The model under review builds one solid part; all positions refer to its coordinate system, in mm. A direction names the side the tool comes from. Give positions to 0.01 mm unless a question says otherwise; leave off trailing zeros. Loops run counter-clockwise (first coordinate to the right, second up) from the corner with the lowest first, then second, coordinate; pieces in that order, holes last. Notation, with made-up numbers: M -30,74.25 L 22,74.25 A30 ccw 22,106.25 Z; hole C 54.25,12 d9. An arc over 180 degrees is marked long. One line per item, written item: value. Start each with the question number.
Q1. We need section C-C on y = 109. Write out the cut boundary in (x, z), plus the area to 3 significant figures.
Q2. For faces 1 (the face through (-1.633, 6.439, -49.684)), 2 (the face through (-0.253, 116.165, -66.719)), 3 (the face through (4, 64, -60.458)), 4 (the face through (-1.633, 112.374, 15.653)), list the 3-axis set-ups (+Z, -Z, +X, -X, +Y, -Y) from which the entire face can be reached by the end or side of a thin tool; tool diameter is ignored.
Q3. For pin 1 (1.5 mm diameter, centred on y = 96.5, z = -54, fed in from +X); pin 2 (2.5 mm diameter, centred on x = -1.03, y = 12.7, fed in from +Z), all flat-tipped, find the tip position at first contact; note any pin that passes through.
Q4. To check wall thickness, follow line 1 along Z through (x, y) = (-2.5, 11.5); line 2 along Y through (x, z) = (2.75, 3); line 3 along X through (y, z) = (114, -67). State the ranges of each line that lie inside material, in increasing order. Write a range as from..to.
Q5. We need section B-B on z = 11. Write out the cut boundary in (x, y).
Q6. We need section A-A on y = 34. Write out the cut boundary in (x, z).
Q7. Mouldability with a two-part tool opening along X and no side actions: class faces 5 (the face through (-1.011, 13.703, -47.408)), 6 (the face through (-1, 63, -73.158)), 7 (the face through (-1.011, 113.95, -59.455)), 8 (the face through (5.323, 68, 10)) as released by +X, released by -X, zero draft, split by the parting line, or undercut.
Autodesk Inventor part; units mm, degrees
ref_plane "YZ Plane" through (0, 0, 0) normal (1, 0, 0) x (0, 1, 0)
ref_plane "XZ Plane" through (0, 0, 0) normal (0, 1, 0) x (-1, 0, 0)
ref_plane "XY Plane" through (0, 0, 0) normal (0, 0, 1) x (1, 0, 0)
sketch "Sketch1" plane through (0, 0, 0) normal (0, 1, 0) x (-1, 0, 0)
  line L0 (7.3766, 22.0919) -> (-5.3234, 22.0919)
  line L1 (-5.3234, 22.0919) -> (-5.3234, -73.1581)
  line L2 (-5.3234, -73.1581) -> (7.3766, -73.1581)
  line L3 (7.3766, -73.1581) -> (7.3766, 22.0919)
  point P0 (0, 0)
  dimension "d0" = 12.7
  dimension "d1" = 95.25
extrude "Extrusion1" add sketch "Sketch1" along normal blind 127
sketch "Sketch2" plane through (-7.3766, 0, 22.0919) normal (0, 0, 1) x (1, 0, 0)
  line L0 (12.7, 0) -> (12.7, 127)
  line L1 (12.7, 127) -> (0, 127)
  line L2 (0, 0) -> (12.7, 0)
  line L3 (0, 0) -> (0, 127)
  point P0 (7.3766, 0)
  point P1 (6.35, 114.3)
  point P2 (6.35, 12.7)
  dimension "d4" = 6.35
  dimension "d5" = 12.7
  dimension "d6" = 12.7
  dimension "d7" = 6.35
hole "Hole1" at (-1.0266, 114.3, 22.0919) at (-1.0266, 12.7, 22.0919) direction (0, 0, -1) diameter 4.0386 depth 12.7 tip angle 118
sketch "Sketch3" plane through (5.3234, 0, -73.1581) normal (0, 0, -1) x (-1, 0, 0)
  line L0 (0, 0) -> (12.7, 0)
  line L1 (12.7, 0) -> (12.7, 127)
  line L2 (0, 127) -> (12.7, 127)
  point P0 (5.3234, 0)
  point P1 (6.35, 114.3)
  point P2 (6.35, 12.7)
  dimension "d15" = 12.7
  dimension "d16" = 6.35
  dimension "d17" = 6.35
  dimension "d18" = 12.7
hole "Hole2" at (-1.0266, 114.3, -73.1581) at (-1.0266, 12.7, -73.1581) direction (0, 0, 1) diameter 4.0386 depth 12.7 tip angle 118
sketch "Sketch4" plane through (5.3234, 0, 22.0919) normal (1, 0, 0) x (0, 0, -1)
  line L0 (12.7, 120.65) -> (82.55, 120.65)
  line L1 (82.55, 120.65) -> (82.55, 6.35)
  line L2 (82.55, 6.35) -> (12.7, 6.35)
  line L3 (12.7, 6.35) -> (12.7, 120.65)
  line L4 (95.25, 127) -> (0, 127)
  line L5 (95.25, 0) -> (0, 0)
  line L6 (95.25, 0) -> (95.25, 127)
  line L7 (0, 0) -> (0, 127)
  point P0 (22.0919, 0)
  dimension "d26" = 6.35
  dimension "d27" = 6.35
  dimension "d28" = 12.7
  dimension "d29" = 12.7
extrude "Extrusion2" cut sketch "Sketch4" against normal blind 3.175 contours L0 L1 L2 L3
sketch "Sketch5" plane through (0, 127, 0) normal (0, 1, 0) x (1, 0, 0)
  line L0 (-7.3766, -22.0919) -> (5.3234, -22.0919)
  line L1 (5.3234, 73.1581) -> (-7.3766, 73.1581)
  line L2 (-7.3766, 73.1581) -> (-7.3766, -22.0919)
  point P0 (0, 0)
  point P1 (-1.0266, 25.5331)
  dimension "d32" = 95.25
  dimension "d33" = 6.35
  dimension "d34" = 47.625
hole "Hole3" at (-1.0266, 127, -25.5331) direction (0, -1, 0) diameter 4.0386 depth 25.4 tip angle 118
sketch "Sketch6" plane through (0, 0, 0) normal (0, -1, 0) x (1, 0, 0)
  line L0 (-7.3766, -73.1581) -> (-7.3766, 22.0919)
  line L1 (-7.3766, 22.0919) -> (5.3234, 22.0919)
  line L2 (5.3234, -73.1581) -> (-7.3766, -73.1581)
  point P0 (0, 0)
  point P1 (-1.0266, -3.3081)
  point P2 (-1.0266, -47.7581)
  dimension "d42" = 6.35
  dimension "d43" = 6.35
  dimension "d44" = 25.4
  dimension "d45" = 25.4
hole "Hole4" at (-1.0266, 0, -3.3081) at (-1.0266, 0, -47.7581) direction (0, 1, 0) diameter 4.0386 depth 12.7 tip angle 118
properties part number "BatteryHighSide"
Solved:
1. outline: M -7.38,-73.16 L 5.32,-73.16 L 5.32,-60.46 L 2.15,-60.46 L 2.15,9.39 L 5.32,9.39 L 5.32,22.09 L -7.38,22.09 Z; hole C -1.03,-25.53 d4.04
1. area: 975 mm2
2. face 1: -Y
2. face 2: -Z
2. face 3: +X
2. face 4: +Z
3. pin 1: x = 2.15
3. pin 2: z = 8.93
4. line 1: -60.39..-49.14, -46.38..-4.69, -1.93..9.32
4. line 2: 0..6.35, 120.65..127
4. line 3: -7.38..-3.02, 0.97..5.32
5. outline: M -7.38,0 L 5.32,0 L 5.32,127 L -7.38,127 Z; hole C -1.03,12.7 d4.04; hole C -1.03,114.3 d4.04
6. outline: M -7.38,-73.16 L 5.32,-73.16 L 5.32,-60.46 L 2.15,-60.46 L 2.15,9.39 L 5.32,9.39 L 5.32,22.09 L -7.38,22.09 Z
7. face 5: undercut
7. face 6: zero draft
7. face 7: undercut
7. face 8: released by +X
